Print and shaded views of the part. All mm, measured from the part's lowest x, y and z. A direction names the side the tool comes from. Round coordinates to 2 decimals unless told otherwise and drop trailing zeros. Write each loop counter-clockwise with the first axis right and the second up, starting at its lowest first coordinate (ties: lowest second). Pieces come first, ordered by that corner, then holes. Notation, with made-up numbers: (7, 4) - (12, 4) arc R18 cw to (12, 25) - close; hole circle Ø9 at (-12.75, -8.5). An arc over 180 degrees is marked (long way). Put each result on its own line as item: value. Start each with the question number.
Item 1: Cut at A-A (z = 15.5). Give the cut face in (x, y).
Item 2: Cut at D-D (x = 9). Give the cut face in (y, z).
Item 3: Drill centre lines: line 1 (X direction, y = 23, z = 18.5); line 2 (Y direction, x = 28, z = 16); line 3 (Y direction, x = 49, z = 12). Where is each one in solid material? Low to high. Write a range as from..to.
Item 4: Pin check, flat tips, straight feed: pin 1 Ø1.5 at (y, z) = (26, 17) entering from +X; pin 2 Ø1.5 at (x, z) = (21.5, 14.5) entering from +Y; pin 3 Ø8 at (x, z) = (36.5, 6) entering from +Y. Stop position of each tip, or through.
Item 5: 3-axis set-ups, long thin cutter, end or side, ignore diameter. For the marked faces 1, 2 and 3: which of +Z, -Z, +X, -X, +Y, -Y reach the whole face in a straight line?
Item 6: Cut at C-C (x = 29.5). Give the cut face in (y, z), and give its area (3 significant figures).
Item 7: Mould opens along Z. For the marked faces 4 and 5 say: released by +Z, released by -Z, zero draft, split by the parting line, or undercut.
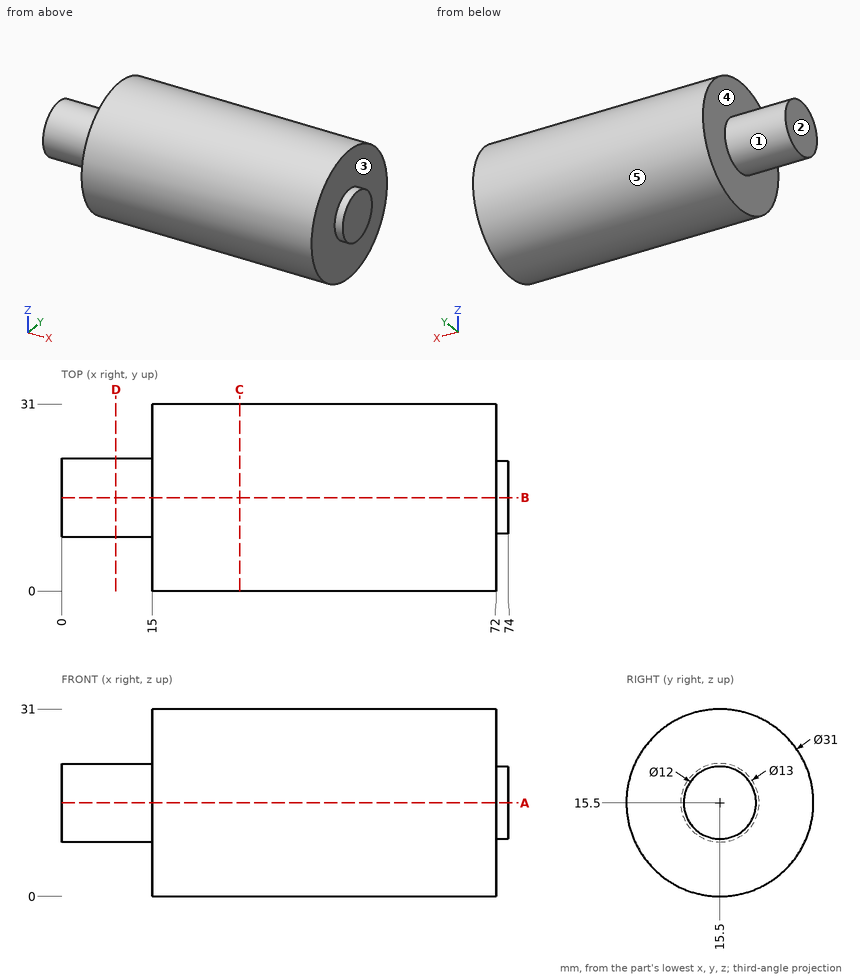
Output values:
1. outline: (0, 9) - (15, 9) - (15, 0) - (72, 0) - (72, 9.5) - (74, 9.5) - (74, 21.5) - (72, 21.5) - (72, 31) - (15, 31) - (15, 22) - (0, 22) - close
2. outline: circle Ø13 at (15.5, 15.5)
3. line 1: 15..72
3. line 2: 0.01..30.99
3. line 3: 0.4..30.6
4. pin 1: x = 72
4. pin 2: y = 31
4. pin 3: y = 29.99
5. face 1: -X
5. face 2: +Z, -Z, -X, +Y, -Y
5. face 3: +X
6. outline: circle Ø31 at (15.5, 15.5)
6. area: 755 mm2
7. face 4: zero draft
7. face 5: split by the parting line
